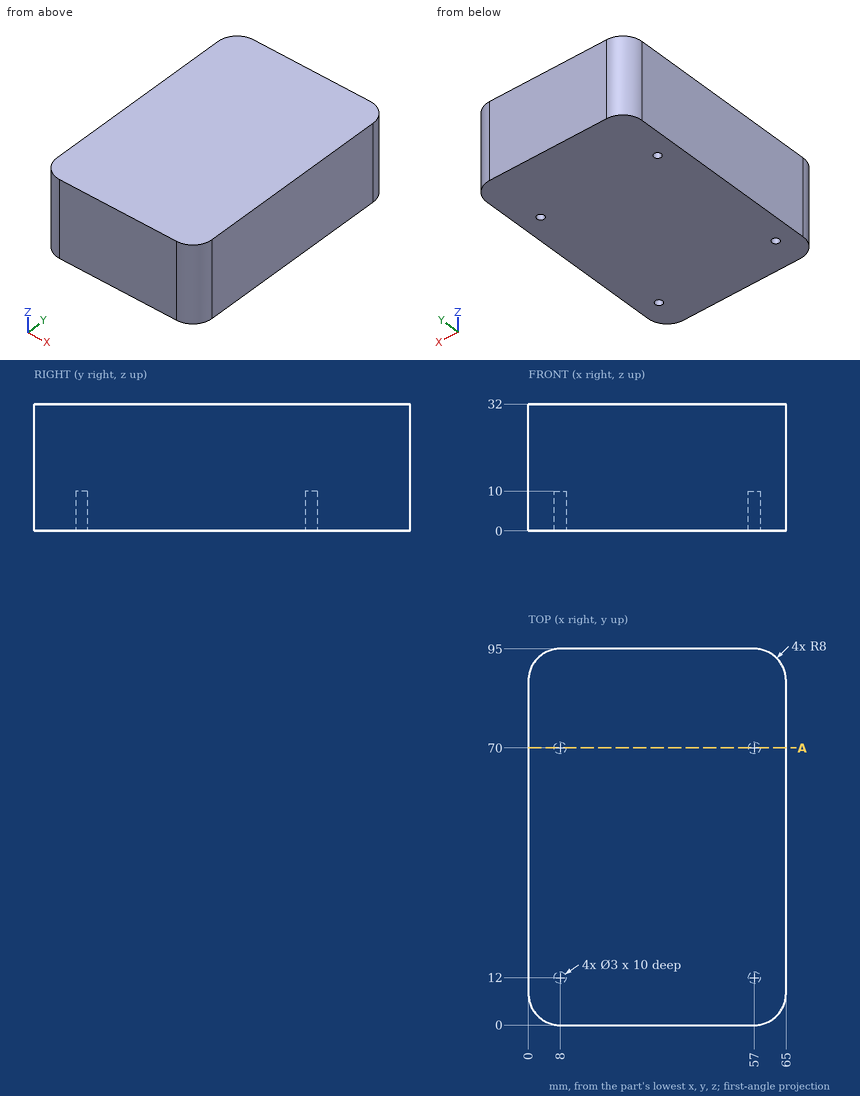
For this review, use the dimensioned drawing (mm, ordinates from the lowest corner) and the shaded views. Round coordinates to 2 decimals unless told otherwise and drop trailing zeros. Order: outer loops, then holes, each group sorted by start corner. A loop starts at its lowest first (then second) coordinate and runs counter-clockwise, first axis right, second up. Notation, with made-up numbers: M 30,-26.75 L 54,-26.75 A31 ccw 54,4.25 Z; hole C -15.75,37 d11. An arc over 180 degrees is marked long. Use a Markdown table: item, result. Add a question column.
Item 1: To check wall thickness, follow line 1 along Y through (x, z) = (8, 4.75); line 2 along X through (y, z) = (70, 6); line 3 along X through (y, z) = (89, 5.5). State the ranges of each line that lie inside material, in increasing order.
Item 2: Add section A-A, the plane y = 70. Give the boundary of the cut face in (x, z), then the cut area to 3 significant figures.
Item 3: Insertion check: pin 1 (3.5 mm diameter, centred on x = 8, y = 70.5, fed in from -Z); pin 2 (1.8 mm diameter, centred on x = 8, y = 70, fed in from -Z). Each pin has a flat end and moves straight along its axis. Give the tip position at first contact, or say it passes through.
Geometry results:
| question | item | result |
|---|---|---|
| 1 | line 1 | y = 0 to 10.5, 13.5 to 68.5, 71.5 to 95 |
| 1 | line 2 | x = 0 to 6.5, 9.5 to 55.5, 58.5 to 65 |
| 1 | line 3 | x = 0.25 to 64.75 |
| 2 | outline | M 0,0 L 6.5,0 L 6.5,10 L 9.5,10 L 9.5,0 L 55.5,0 L 55.5,10 L 58.5,10 L 58.5,0 L 65,0 L 65,32 L 0,32 Z |
| 2 | area | 2,020 mm² |
| 3 | pin 1 | stops at z = 0 |
| 3 | pin 2 | stops at z = 10 |
